Autodesk Inventor part; units mm, degrees
ref_plane "Work Plane1" through (-7.5, 0, 0) normal (1, 0, 0) x (0, 1, 0)
ref_plane "Work Plane2" through (-4.25, 0, 0) normal (1, 0, 0) x (0, 1, 0)
ref_plane "Work Plane3" through (0, 9, 0) normal (0, 1, 0) x (1, 0, 0)
sketch "Sketch1" plane through (0, 0, 0) normal (0, 1, 0) x (-1, 0, 0)
  line L0 (0, 0) -> (15, 0)
  line L1 (15, 0) -> (15, 120)
  line L2 (15, 120) -> (0, 120)
  line L3 (0, 120) -> (0, 0)
  dimension "d0" = 15
  dimension "d1" = 120
extrude "Extrusion1" add sketch "Sketch1" along normal blind 3
sketch "Sketch3" plane through (0, 0, 120) normal (1, 0, 0) x (0, 0, -1)
  line L0 (120, 0) -> (115, 0)
  line L1 (0, 0) -> (120, 0)
  line L2 (115, 0) -> (115, 3)
  line L3 (0, 3) -> (120, 3)
  line L4 (115, 3) -> (115, 13)
  line L5 (120, 13) -> (120, 3)
  line L6 (120, 3) -> (115, 3)
  arc A0 (120, 13) -> (115, 13) centre (117.5, 13) ccw
  dimension "d4" = 5
  dimension "d5" = 10
extrude "Extrusion2" add sketch "Sketch3" against normal blind 2
ref_plane "Work Plane1" through (-7.5, 0, 0) normal (1, 0, 0) x (0, 1, 0)
mirror "Mirror1" about plane through (-7.5, 0, 0) normal (1, 0, 0) of "Extrusion2"
ref_plane "Work Plane2" through (-4.25, 0, 0) normal (1, 0, 0) x (0, 1, 0)
mirror "Mirror2" about plane through (-4.25, 0, 0) normal (1, 0, 0) of "Extrusion2"
sketch "Sketch6" plane through (-6.5, 3, 0) normal (1, 0, 0) x (0, 0, -1)
  line L0 (0, 0) -> (-5, 0)
  line L1 (-5, 0) -> (-5, 10)
  line L2 (-5, 0) -> (-5, 10)
  line L3 (-5, 10) -> (-5, 0)
  arc A0 (0, 10) -> (-5, 10) centre (-2.5, 10) ccw
  arc A1 (0, 10) -> (-5, 10) centre (-2.5, 10) ccw
  line L4 (0, 10) -> (0, 0)
  line L5 (0, 10) -> (0, 0)
  point P0 (0, -3)
extrude "Extrusion3" add sketch "Sketch6" along normal blind 2
mirror "Mirror3" about plane through (-7.5, 0, 0) normal (1, 0, 0) of "Extrusion3"
sketch "Sketch9" plane through (0, 0, 120) normal (1, 0, 0) x (0, 0, -1)
  line L0 (120, 0) -> (75, 0)
  line L1 (120, 0) -> (0, 0)
  line L2 (75, 0) -> (75, 3)
  line L3 (0, 3) -> (115, 3)
  line L4 (75, 3) -> (72, 3)
  line L5 (75, 3) -> (78, 3)
  line L6 (75, 3) -> (75, 6)
  circle A0 centre (75, 6) radius 1.5
  line L7 (72, 3) -> (72, 6)
  line L8 (78, 3) -> (78, 6)
  arc A1 (78, 6) -> (72, 6) centre (75, 6) ccw
  dimension "d16" = 45
  dimension "d17" = 3
  dimension "d18" = 3
  dimension "d20" = 3
extrude "Extrusion4" add sketch "Sketch9" against normal blind 2
mirror "Mirror4" about plane through (-7.5, 0, 0) normal (1, 0, 0) of "Extrusion4"
mirror "Mirror5" about plane through (-4.25, 0, 0) normal (1, 0, 0) of "Extrusion4"
sketch "Sketch10" plane through (-6.5, 3, 42) normal (1, 0, 0) x (0, 0, -1)
  line L0 (-6, 0) -> (0, 0)
  line L1 (0, 0) -> (-6, 0)
  line L2 (0, 0) -> (0, 3)
  arc A0 (0, 3) -> (-6, 3) centre (-3, 3) ccw
  arc A1 (0, 3) -> (-6, 3) centre (-3, 3) ccw
  line L3 (-6, 0) -> (-6, 3)
  line L4 (-6, 0) -> (-6, 3)
  point P0 (42, -3)
extrude "Extrusion5" add sketch "Sketch10" along normal blind 2
sketch "Sketch11" plane through (-6.5, 6, 45) normal (-1, 0, 0) x (0, 0, 1)
  circle A0 centre (0, 0) radius 1.5
  point P0 (-45, -6)
extrude "Extrusion6" cut sketch "Sketch11" against normal blind 2
mirror "Mirror6" about plane through (-7.5, 0, 0) normal (1, 0, 0) of "Extrusion5", "Extrusion6"
sketch "Sketch12" plane through (0, 3, 0) normal (0, 1, 0) x (1, 0, 0)
  line L0 (0, -120) -> (-15, -120)
  line L1 (-15, -120) -> (-15, -48)
  line L2 (-15, -48) -> (0, -48)
  line L3 (0, -48) -> (0, -120)
  point P0 (0, 0)
extrude "Extrusion7" cut sketch "Sketch12" against normal blind 3
sketch "Sketch13" plane through (0, 3, 0) normal (0, 1, 0) x (1, 0, 0)
  line L0 (-15, -5) -> (-15, -42)
  line L1 (-15, -42) -> (-13, -42)
  line L2 (-15, -42) -> (-13, -42)
  line L3 (-13, -42) -> (-13, -48)
  line L4 (-13, -42) -> (-13, -48)
  line L5 (-13, -48) -> (-10.5, -48)
  line L6 (-10.5, -48) -> (-10.5, -42)
  line L7 (-10.5, -48) -> (-10.5, -42)
  line L8 (-10.5, -42) -> (-4.5, -42)
  line L9 (-10.5, -42) -> (-4.5, -42)
  line L10 (-4.5, -42) -> (-4.5, -48)
  line L11 (-4.5, -48) -> (-2, -48)
  line L12 (-4.5, -48) -> (-2, -48)
  line L13 (-2, -48) -> (-2, -42)
  line L14 (-2, -48) -> (-2, -42)
  line L15 (-2, -42) -> (0, -42)
  line L16 (0, -42) -> (0, -5)
  line L17 (0, -5) -> (-2, -5)
  line L18 (-2, -5) -> (-2, 0)
  line L19 (-2, 0) -> (-4.5, 0)
  line L20 (-4.5, 0) -> (-4.5, -5)
  line L21 (-4.5, -5) -> (-10.5, -5)
  line L22 (-4.5, -5) -> (-10.5, -5)
  line L23 (-10.5, -5) -> (-10.5, 0)
  line L24 (-10.5, 0) -> (-13, 0)
  line L25 (-10.5, 0) -> (-13, 0)
  line L26 (-13, 0) -> (-13, -5)
  line L27 (-13, -5) -> (-15, -5)
  line L28 (-13, -5) -> (-15, -5)
  line L29 (-15, -5) -> (-15, -42)
  line L30 (-15, 0) -> (-15, -48)
  point P0 (0, 0)
extrude "Extrusion8" cut sketch "Sketch13" against normal blind 1
ref_plane "Work Plane3" through (0, 9, 0) normal (0, 1, 0) x (1, 0, 0)
sketch "Sketch15" plane through (0, 9, 0) normal (0, 1, 0) x (1, 0, 0)
  line L0 (-4.5, -48) -> (-4.5, -42)
  line L1 (-4.5, -45) -> (-10.5, -45)
  line L2 (-10.5, -48) -> (-10.5, -42)
  circle A0 centre (-7.5, -45) radius 0.8
  point P0 (0, 0)
  dimension "d32" = 1.6
extrude "Extrusion9" cut sketch "Sketch15" against normal blind 3
properties part number "armholder"
Geometry: final body of the model. Coordinates: model frame, mm. A direction names the side the tool comes from. Round coordinates to 2 decimals unless told otherwise and drop trailing zeros. Order: outer loops, then holes, each group sorted by start corner. A loop starts at its lowest first (then second) coordinate and runs counter-clockwise, first axis right, second up. Notation, with made-up numbers: (59.5, 40.25) -> (107.5, 40.25) arc R38 cw to (107.5, 79.25) -> close; hole circle Ø3 at (27.25, -23). An arc over 180 degrees is marked (long way). Use one line per item in the form item = value.
(1) Section C-C on z = 45. Return loops of the section in (x, y), and give its area (3 significant figures).
Results list:
outline = (-15, 0) -> (0, 0) -> (0, 4.5) -> (-2, 4.5) -> (-2, 2) -> (-4.5, 2) -> (-4.5, 4.5) -> (-10.5, 4.5) -> (-10.5, 2) -> (-13, 2) -> (-13, 4.5) -> (-15, 4.5) -> close; (-15, 7.5) -> (-13, 7.5) -> (-13, 9) -> (-15, 9) -> close; (-10.5, 7.5) -> (-8.3, 7.5) -> (-8.3, 9) -> (-10.5, 9) -> close; (-6.7, 7.5) -> (-4.5, 7.5) -> (-4.5, 9) -> (-6.7, 9) -> close; (-2, 7.5) -> (0, 7.5) -> (0, 9) -> (-2, 9) -> close
area = 67.6 mm^2
(2) Access query for faces 1 (the face through (-1, 8, 5)), 2 (the face through (-10.5, 4, 45)), 3 (the face through (-7, 6, 0)). Directions: +Z, -Z, +X, -X, +Y, -Y. A direction counts if a zero-diameter tool reaches every point of the face in a straight line with its end or side. Return the directions, or none.
Results list:
face_1 = +X, -X, +Y
face_2 = +Z, -Z, +Y
face_3 = -Z, +X, -X, +Y, -Y
(3) Section A-A on y = 4. Return loops of the section in (x, z), and give its area (3 significant figures).
Results list:
outline = (-15, 0) -> (-13, 0) -> (-13, 5) -> (-15, 5) -> close; (-15, 42) -> (-13, 42) -> (-13, 48) -> (-15, 48) -> close; (-10.5, 0) -> (-4.5, 0) -> (-4.5, 5) -> (-10.5, 5) -> close; (-10.5, 42) -> (-4.5, 42) -> (-4.5, 48) -> (-10.5, 48) -> close; (-2, 0) -> (0, 0) -> (0, 5) -> (-2, 5) -> close; (-2, 42) -> (0, 42) -> (0, 48) -> (-2, 48) -> close
area = 110 mm^2
(4) Section D-D on y = 11.5. Return loops of the section in (x, z).
Results list:
outline = (-15, 0) -> (-13, 0) -> (-13, 5) -> (-15, 5) -> close; (-10.5, 0) -> (-4.5, 0) -> (-4.5, 5) -> (-10.5, 5) -> close; (-2, 0) -> (0, 0) -> (0, 5) -> (-2, 5) -> close
(5) Ray query, probe 1 along Z at (x, y) = (-0.95, 6); probe 2 along Y at (x, z) = (-5.1, 45); probe 3 along X at (y, z) = (7.7, 45). Return the intervals inside material, ascending. Write a range as [from, to].
Results list:
probe_1 = [0, 5], [42, 43.5], [46.5, 48]
probe_2 = [0, 4.5], [7.5, 9]
probe_3 = [-15, -13], [-10.5, -8.3], [-6.7, -4.5], [-2, 0]
(6) First-contact query: pin 1 Ø1.4 at (x, z) = (-7.5, 45) entering from +Y; pin 2 Ø2.5 at (y, z) = (8.5, 1.5) entering from +X; pin 3 Ø2.5 at (y, z) = (6, 45) entering from +X; pin 4 Ø1.5 at (x, z) = (-13, 18.5) entering from +Y. Flat tips, straight axial feed; report the tip coordinate or a pass-through.
Results list:
pin_1 = 4.67
pin_2 = 0
pin_3 = through
pin_4 = 2
(7) Section B-B on x = -9. Return loops of the section in (y, z), and give its area (3 significant figures).
Results list:
outline = (0, 0) -> (13, 0) arc R2.5 ccw to (13, 5) -> (2, 5) -> (2, 42) -> (6, 42) arc R3 ccw to (6, 48) -> (0, 48) -> close; hole circle Ø3 at (6, 45)
area = 192 mm^2
(8) Draft query along X for faces 4 (the face through (-15, 1, 20)), 5 (the face through (-7, 2, 48)), 6 (the face through (-4.5, 4, 45)). Return one class per face: pulls with the +X half, pulls with the -X half, needs draft (parallel to the pull), parting line crosses it, or undercut.
Results list:
face_4 = pulls with the -X half
face_5 = needs draft
face_6 = undercut
